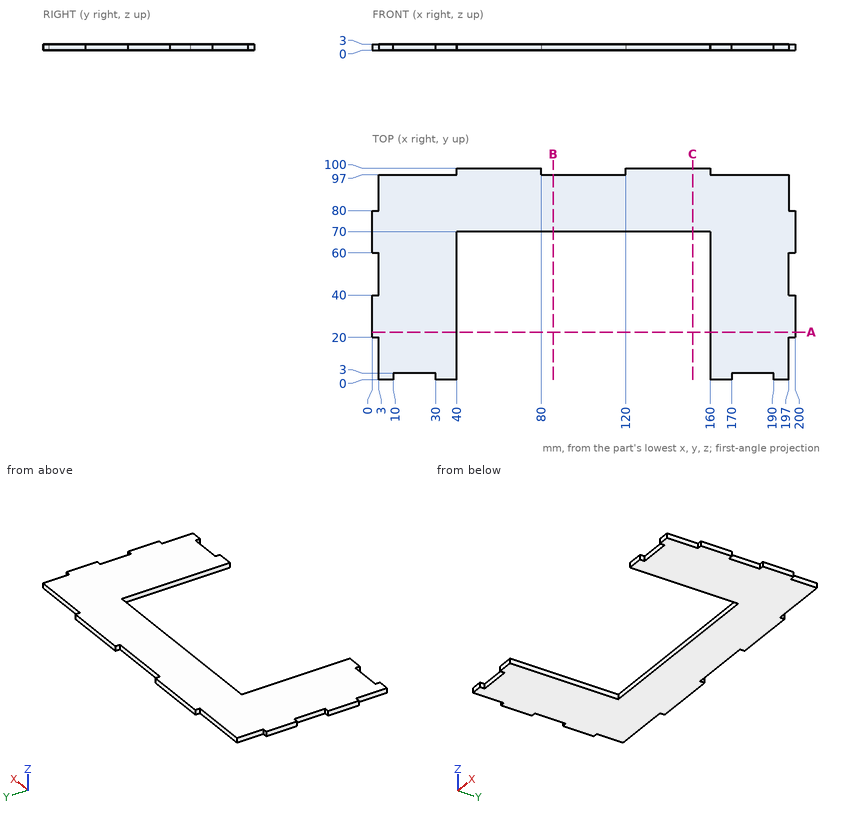
Study the drawing (mm; zero at the part's minimum x, y, z) and answer. Give positions to 0.01 mm unless a question says otherwise; leave off trailing zeros. Loops run counter-clockwise (first coordinate to the right, second up) from the corner with the lowest first, then second, coordinate; pieces in that order, holes last. Notation, with made-up numbers: (84, 52.5) - (136, 52.5) arc R25 ccw to (136, 67.5) - close; hole circle Ø11 at (-38.75, 54.5). An arc over 180 degrees is marked (long way). Return JSON: item names as keys, results as strings. Group by question number.
1. Straight lines are drawn through the part: line 1 (X direction, y = 18.5, z = 0.75); line 2 (X direction, y = 25, z = 2.6); line 3 (Y direction, x = 158, z = 0.6). For each, find the intervals that lie inside material, in ascending order. Write a range as [from, to].
2. Find section B-B (x = 85.5). Write down the section's boundary in (y, z).
3. Find section A-A (y = 22.5). Write down the section's boundary in (x, z).
4. Find section C-C (x = 151.5). Write down the section's boundary in (y, z).
5. Given pin 1 Ø1.5 at (x, z) = (1, 2) entering from -Y; pin 2 Ø1.5 at (y, z) = (8.5, 1.5) entering from -X; pin 3 Ø0.9 at (y, z) = (99, 1) entering from +X, each flat-ended and moving along its own axis, determine where each tip first touches the part or whether it passes through.
Verdict:
{
 "1": {"line 1": "x = [3, 40], [160, 197]", "line 2": "x = [0, 40], [160, 200]", "line 3": "y = [70, 100]"},
 "2": {"outline": "(70, 0) - (97, 0) - (97, 3) - (70, 3) - close"},
 "3": {"outline": "(0, 0) - (40, 0) - (40, 3) - (0, 3) - close; (160, 0) - (200, 0) - (200, 3) - (160, 3) - close"},
 "4": {"outline": "(70, 0) - (100, 0) - (100, 3) - (70, 3) - close"},
 "5": {"pin 1": "stops at y = 20", "pin 2": "stops at x = 3", "pin 3": "stops at x = 160"}
}
